Input: part model. Units: mm. Frame: model coordinates. Round coordinates to 2 decimals unless told otherwise and drop trailing zeros. Loops run counter-clockwise (first coordinate to the right, second up) from the corner with the lowest first, then second, coordinate; pieces in that order, holes last. Notation, with made-up numbers: (81.5, 14.25) -> (103.5, 14.25) arc R21 ccw to (103.5, 22.25) -> close; hole circle Ø2 at (13, 61). An arc over 180 degrees is marked (long way). Answer as a JSON object with one key per item and string values.
```python
from build123d import *

# Parameters (mm, degrees)
BASE_FLANGE1_DEPTH  = 0.7
BREAK_CORNER1_START = -0.7
BREAK_CORNER1_DEPTH = 0.7


# Read off the part's stored shape, not the designer's step: Break-Corner1
# Sheet-metal steps are written as plain solids
with BuildPart() as part:
    # Sketch1 → Base-Flange1 (new body)
    with BuildSketch(Plane.XY):
        Polygon((0, 0), (0, 30), (30, 0), align=None)
    extrude(amount=-BASE_FLANGE1_DEPTH)

    # Break-Corner1 outline → Break-Corner1 (cut)
    with BuildSketch(Plane.XY.offset(BREAK_CORNER1_START)):
        with BuildLine():
            ThreePointArc((2.499, 0), (0.731940154, 0.731940154), (0, 2.499))
            Line((0, 2.499), (0, 0))
            Line((0, 0), (2.499, 0))
        make_face()
        with BuildLine():
            Line((0, 30), (0, 23.966880308))
            ThreePointArc((0, 23.966880308), (1.542674103, 26.275655259), (4.266059846, 25.733940154))
            Line((4.266059846, 25.733940154), (0, 30))
        make_face()
        with BuildLine():
            ThreePointArc((25.733940154, 4.266059846), (26.275655259, 1.542674103), (23.966880308, 0))
            Line((23.966880308, 0), (30, 0))
            Line((30, 0), (25.733940154, 4.266059846))
        make_face()
    extrude(amount=BREAK_CORNER1_DEPTH, mode=Mode.SUBTRACT)


solid = part.part
```
1) Ray query, probe 1 along Y at (x, z) = (7.5, -0.2); probe 2 along Y at (x, z) = (15.25, -0.45); probe 3 along X at (y, z) = (22.25, -0.15). Return the intervals inside material, ascending.
Output:
{"probe 1": "y = 0 to 22.5", "probe 2": "y = 0 to 14.75", "probe 3": "x = 0 to 7.75"}
2) Section C-C, the plane y = 23.25. Output: boundary loops of the cut face in (x, z), plus the area to 4 significant figures.
Output:
{"outline": "(0, -0.7) -> (6.75, -0.7) -> (6.75, 0) -> (0, 0) -> close", "area": "4.725 mm^2"}
3) Section A-A, the plane z = -0.55. Output: boundary loops of the cut face in (x, y), plus the area to 3 significant figures.
Output:
{"outline": "(0, 2.5) arc R2.5 ccw to (2.5, 0) -> (23.97, 0) arc R2.5 ccw to (25.73, 4.27) -> (4.27, 25.73) arc R2.5 ccw to (0, 23.97) -> close", "area": "433 mm^2"}
4) Section B-B, the plane x = 21. Output: boundary loops of the cut face in (y, z), plus the area to 3 significant figures.
Output:
{"outline": "(0, -0.7) -> (9, -0.7) -> (9, 0) -> (0, 0) -> close", "area": "6.30 mm^2"}
